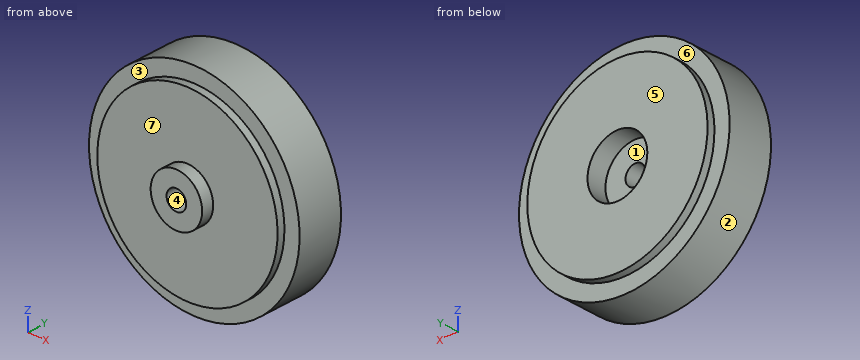
```python
from build123d import *

# Parameters (mm, degrees)
SKETCH1_R           = 69.5
BOSS_EXTRUDE1_DEPTH = 40
CUT_EXTRUDE1_START  = -5
SKETCH2_R           = 69.5
SKETCH2_R_2         = 59.5
CUT_EXTRUDE1_DEPTH  = 5
SKETCH3_R           = 69.5
SKETCH3_R_2         = 59.5
CUT_EXTRUDE2_DEPTH  = 5
SKETCH4_R           = 19.75
CUT_EXTRUDE4_DEPTH  = 13
SKETCH5_R           = 17
BOSS_EXTRUDE2_DEPTH = 8
SKETCH6_R           = 6.5
CUT_EXTRUDE5_DEPTH  = 110.382356895


with BuildPart() as part:
    # Sketch1 → Boss-Extrude1 (new body)
    with BuildSketch(Plane(origin=(0, 0, 0), x_dir=(1, 0, 0), z_dir=(0, 1, 0))):
        with Locations(Location((0, 0, 0), (0, 0, 270))):
            Circle(SKETCH1_R)
    extrude(amount=BOSS_EXTRUDE1_DEPTH)

    # Sketch2 → Cut-Extrude1 (cut)
    with BuildSketch(Plane(origin=(0, 40, 0), x_dir=(1, 0, 0), z_dir=(0, 1, 0)).offset(CUT_EXTRUDE1_START)):
        with Locations(Location((0, 0, 0), (0, 0, 270))):
            Circle(SKETCH2_R)
        with Locations(Location((0, 0, 0), (0, 0, 270))):
            Circle(SKETCH2_R_2, mode=Mode.SUBTRACT)
    extrude(amount=CUT_EXTRUDE1_DEPTH, mode=Mode.SUBTRACT)

    # Sketch3 → Cut-Extrude2 (cut)
    with BuildSketch(Plane.XZ):
        with Locations(Location((0, 0, 0), (0, 0, 270))):
            Circle(SKETCH3_R)
        with Locations(Location((0, 0, 0), (0, 0, 90))):
            Circle(SKETCH3_R_2, mode=Mode.SUBTRACT)
    extrude(amount=-CUT_EXTRUDE2_DEPTH, mode=Mode.SUBTRACT)

    # Sketch4 → Cut-Extrude4 (cut)
    with BuildSketch(Plane(origin=(0, 40, 0), x_dir=(1, 0, 0), z_dir=(0, 1, 0))):
        with Locations(Location((0, 0, 0), (0, 0, 270))):
            Circle(SKETCH4_R)
    extrude(amount=-CUT_EXTRUDE4_DEPTH, mode=Mode.SUBTRACT)

    # Sketch5 → Boss-Extrude2 (add)
    with BuildSketch(Plane.XZ):
        with Locations(Location((0, 0, 0), (0, 0, 270))):
            Circle(SKETCH5_R)
    extrude(amount=BOSS_EXTRUDE2_DEPTH)

    # Sketch6 → Cut-Extrude5 (cut, through all)
    with BuildSketch(Plane.XZ.offset(8)):
        with Locations(Location((0, 0, 0), (0, 0, 270))):
            Circle(SKETCH6_R)
    extrude(amount=-CUT_EXTRUDE5_DEPTH, mode=Mode.SUBTRACT)


solid = part.part
```
Work out the finished part from the listing and answer in its coordinate system (mm). Face numbers are marked on the shaded views. A direction names the side the tool comes from. Give positions to 0.01 mm unless a question says otherwise; leave off trailing zeros. Loops run counter-clockwise (first coordinate to the right, second up) from the corner with the lowest first, then second, coordinate; pieces in that order, holes last. Notation, with made-up numbers: (-21.5, 89) -> (1.5, 89) arc R34 ccw to (1.5, 123) -> close; hole circle Ø3 at (48, 38). An arc over 180 degrees is marked (long way). One line per question, with ' | ' between items. Start each with the question number.
1) Determine the mould class of the marked faces 1, 2, 3 and 4 for opening direction Z: +Z half, -Z half, draft (parallel to the pull), parting line (faces both ways), or undercut.
2) Section C-C, the plane y = 22.5 is taken. Determine the outline of the cut face in (x, z), then the cut area to 3 significant figures.
3) Straight lines are drawn through the part: L1, parallel to X at y = 4, z = 0; L2, parallel to X at y = 34, z = 0; L3, parallel to Y at x = -18, z = -19. For each, find the intervals that lie inside material, in ascending order.
4) Each of these flat-tipped pins is pushed along its axis until it touches: pin 1 (10 mm diameter, centred on y = 20.5, z = 30.5, fed in from -X); pin 2 (2 mm diameter, centred on y = 31, z = -24, fed in from -X); pin 3 (12 mm diameter, centred on x = 6.5, z = 6, fed in from +Y). Where does it stop, or does it pass through?
5) Section A-A, the plane x = 0 is taken. Determine the outline of the cut face in (y, z), then the cut area to 3 significant figures.
6) Section B-B, the plane z = 0 is taken. Determine the outline of the cut face in (x, y).
7) For the marked faces 5, 6 and 7, determine the directions among +Z, -Z, +X, -X, +Y, -Y from which every point of the face is accessible in a straight line to the end or side of a thin tool.
8) Section D-D, the plane x = 45 is taken. Determine the outline of the cut face in (y, z).
Resolved:
1) face 1: undercut | face 2: parting line | face 3: draft | face 4: undercut
2) outline: circle Ø139 at (0, 0); hole circle Ø13 at (0, 0) | area: 15,000 mm2
3) L1: -59.5 to -6.5, 6.5 to 59.5 | L2: -69.5 to -19.75, 19.75 to 69.5 | L3: 0 to 40
4) pin 1: x = -64.65 | pin 2: x = -65.58 | pin 3: y = 27
5) outline: (-8, -17) -> (0, -17) -> (0, -59.5) -> (5, -59.5) -> (5, -69.5) -> (35, -69.5) -> (35, -59.5) -> (40, -59.5) -> (40, -19.75) -> (27, -19.75) -> (27, -6.5) -> (-8, -6.5) -> close; (-8, 6.5) -> (27, 6.5) -> (27, 19.75) -> (40, 19.75) -> (40, 59.5) -> (35, 59.5) -> (35, 69.5) -> (5, 69.5) -> (5, 59.5) -> (0, 59.5) -> (0, 17) -> (-8, 17) -> close | area: 4,660 mm2
6) outline: (-69.5, 5) -> (-59.5, 5) -> (-59.5, 0) -> (-17, 0) -> (-17, -8) -> (-6.5, -8) -> (-6.5, 27) -> (-19.75, 27) -> (-19.75, 40) -> (-59.5, 40) -> (-59.5, 35) -> (-69.5, 35) -> close; (6.5, -8) -> (17, -8) -> (17, 0) -> (59.5, 0) -> (59.5, 5) -> (69.5, 5) -> (69.5, 35) -> (59.5, 35) -> (59.5, 40) -> (19.75, 40) -> (19.75, 27) -> (6.5, 27) -> close
7) face 5: +Z, -Z, +X, -X, +Y | face 6: +Y | face 7: -Y
8) outline: (0, -38.93) -> (5, -38.93) -> (5, -52.96) -> (35, -52.96) -> (35, -38.93) -> (40, -38.93) -> (40, 38.93) -> (35, 38.93) -> (35, 52.96) -> (5, 52.96) -> (5, 38.93) -> (0, 38.93) -> close
